CAD build for the part. Positions are in the model's coordinates, mm. Face numbers are marked on the shaded views. A direction names the side the tool comes from. Round coordinates to 2 decimals unless told otherwise and drop trailing zeros. Loops run counter-clockwise (first coordinate to the right, second up) from the corner with the lowest first, then second, coordinate; pieces in that order, holes last. Notation, with made-up numbers: M -1,24 L 25,24 A36 ccw 25,62 Z; hole C -39,87.25 d10. An arc over 180 degrees is marked long. Use one line per item in the form item = value.
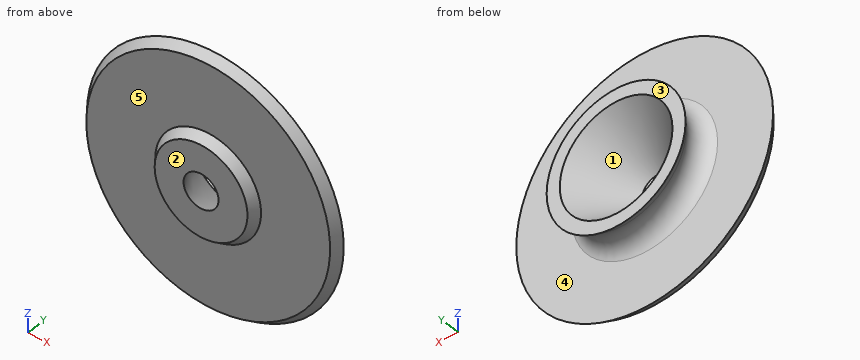
from build123d import *


with BuildPart() as part:
    # Sketch1 → Revolve1 (revolve)
    with BuildSketch(Plane.XY):
        with BuildLine():
            Line((-0.915133072, -47.682722084), (-21.935744519, -47.682722084))
            Line((-21.935744519, -47.682722084), (-26.646227047, -41.332722084))
            Line((-26.646227047, -41.332722084), (-76.783206885, -41.332722084))
            Line((-76.783206885, -41.332722084), (-81.493689413, -34.982722084))
            Line((-81.493689413, -34.982722084), (-41.186438296, -34.982722084))
            ThreePointArc((-41.186438296, -34.982722084), (-32.688024732, -26.842579107), (-34.522388815, -15.218463262))
            Line((-34.522388815, -15.218463262), (-38.70302824, -9.582722084))
            Line((-38.70302824, -9.582722084), (-29.17802824, -9.582722084))
            Line((-29.17802824, -9.582722084), (-0.915133072, -47.682722084))
        make_face()
    revolve(axis=Axis((11.784866928, -49.703724191, 0), (0, 1, 0)))


solid = part.part
1. Cut at B-B on y = -28.5. Write the cut outline in (x, z), and give its area (3 significant figures).
Completed:
outline = C 11.78,0 d90.33; hole C 11.78,0 d53.86
area = 4,130 mm2
2. Pull direction Z, two halves, no side cores. Call the marked faces 1 and 2: +Z half, -Z half, draft (parallel to the pull), parting line (faces both ways), or undercut.
Completed:
face_1 = undercut
face_2 = draft
3. Cut at A-A on z = 0. Write the cut outline in (x, y), and give its area (3 significant figures).
Completed:
outline = M -81.49,-34.98 L -76.78,-41.33 L -26.65,-41.33 L -21.94,-47.68 L -0.92,-47.68 L -29.18,-9.58 L -38.7,-9.58 L -34.52,-15.22 A12.7 cw -41.19,-34.98 Z; M 24.48,-47.68 L 45.51,-47.68 L 50.22,-41.33 L 100.35,-41.33 L 105.06,-34.98 L 64.76,-34.98 A12.7 cw 58.09,-15.22 L 62.27,-9.58 L 52.75,-9.58 Z
area = 1,920 mm2
4. Probe line 1 along Y through (x, z) = (-48, -19.5); line 2 along Z through (x, y) = (29.5, -15.5); line 3 along Z through (x, y) = (9.5, -30). List the from-to ranges inside material, lowest first. Write a range as from..to.
Completed:
line_1 = -41.33..-34.98
line_2 = -42.57..-32, 32..42.57
line_3 = -46..-25.72, 25.72..46
5. Drop flat-ended pins along their axis: P1, Ø12, axis at y = -43.5, z = -71.5, coming from the +X side; P2, Ø2, axis at y = -32, z = -36, coming from the -X side; P3, Ø3, axis at x = 34.5, y = -27, coming from the -Z side; P4, Ø8, axis at x = -0.5, z = 35, coming from the -Y side. Give the stop position or say it passes through.
Completed:
P1 = 71.75
P2 = -21.68
P3 = -39.4
P4 = -47.68
6. Tool access for the marked faces 3, 4 and 5: list every direction of +Z, -Z, +X, -X, +Y, -Y with a clear straight run to the whole face (end or side of a thin tool).
Completed:
face_3 = +Z, -Z, +X, -X, +Y
face_4 = +Y
face_5 = -Y
